from build123d import *

# Parameters (mm, degrees)
SKETCH1_W               = 177.8
SKETCH1_H               = 25.4
BOSS_EXTRUDE1_DEPTH     = 4.826
SKETCH2_W               = 46.566666667
SKETCH2_H               = 4.826
SKETCH2_W_2             = 46.566666666
BOTTOM_EDGE_SLOTS_DEPTH = 180.669948172
SKETCH3_W               = 79.375
SKETCH3_H               = 4.826
TOP_EDGE_SLOTS_DEPTH    = 180.669948172
SKETCH4_W               = 4.826
SKETCH4_H               = 15.748
EDGE_CUTS_DEPTH         = 180.669948172


with BuildPart() as part:
    # Sketch1 → Boss-Extrude1 (new body)
    with BuildSketch(Plane.XY):
        with Locations((88.9, 12.7)):
            Rectangle(SKETCH1_W, SKETCH1_H)
    extrude(amount=BOSS_EXTRUDE1_DEPTH)

    # Sketch2 → Bottom Edge Slots (cut, through all)
    with BuildSketch(Plane.XY.offset(4.826)):
        with Locations((23.283333333, 2.413)):
            Rectangle(SKETCH2_W, SKETCH2_H)
        with Locations((88.9, 2.413)):
            Rectangle(SKETCH2_W_2, SKETCH2_H)
        with Locations((154.516666667, 2.413)):
            Rectangle(SKETCH2_W, SKETCH2_H)
    extrude(amount=-BOTTOM_EDGE_SLOTS_DEPTH, mode=Mode.SUBTRACT)

    # Sketch3 → Top Edge Slots (cut, through all)
    with BuildSketch(Plane.XY.offset(4.826)):
        with Locations((39.6875, 22.987)):
            Rectangle(SKETCH3_W, SKETCH3_H)
        with Locations((138.1125, 22.987)):
            Rectangle(SKETCH3_W, SKETCH3_H)
    extrude(amount=-TOP_EDGE_SLOTS_DEPTH, mode=Mode.SUBTRACT)

    # Sketch4 → Edge Cuts (cut, through all)
    with BuildSketch(Plane.XY.offset(4.826)):
        with Locations((2.413, 12.7)):
            Rectangle(SKETCH4_W, SKETCH4_H)
        with Locations((175.387, 12.7)):
            Rectangle(SKETCH4_W, SKETCH4_H)
    extrude(amount=-EDGE_CUTS_DEPTH, mode=Mode.SUBTRACT)


solid = part.part
Design review of the part built by this model. Coordinates are the model's own, in mm. A direction names the side the tool comes from. Give positions to 0.01 mm unless a question says otherwise; leave off trailing zeros. Order: outer loops, then holes, each group sorted by start corner. A loop starts at its lowest first (then second) coordinate and runs counter-clockwise, first axis right, second up.
1. Mouldability with a two-part tool opening along X and no side actions: class faces 1 (the flat face through (131.233, 2, 2)), 2 (the flat face through (56, 0, 2)), 3 (the flat face through (65.617, 2, 2)) as +X half, -X half, draft (parallel to the pull), parting line (faces both ways), or undercut.
Solution:
face 1: +X half
face 2: draft
face 3: undercut
2. Add section C-C, the plane y = 23.25. State the section outline as (x, z) points (3 decimals), then the cut area to 3 significant figures.
Solution:
outline: (79.375, 0) - (98.425, 0) - (98.425, 4.826) - (79.375, 4.826) - close
area: 91.9 mm2
3. To check wall thickness, follow L1, parallel to X at y = 4.25, z = 0.4; L2, parallel to Y at x = 128.5, z = 0.2; L3, parallel to Y at x = 22, z = 2.75. State the ranges of each line that lie inside material, in increasing order.
Solution:
L1: x = 46.57 to 65.62, 112.18 to 131.23
L2: y = 0 to 20.57
L3: y = 4.83 to 20.57
4. Add section B-B, the plane x = 101. State the section outline as (y, z) points, then the cut area to 3 significant figures.
Solution:
outline: (4.83, 0) - (20.57, 0) - (20.57, 4.83) - (4.83, 4.83) - close
area: 76.0 mm2
5. For pin 1 Ø4 at (x, y) = (105, 17.5) entering from -Z; pin 2 Ø1.4 at (x, z) = (143.5, 3) entering from +Y; pin 3 Ø2.5 at (y, z) = (1.5, 1.5) entering from -X; pin 4 Ø1.4 at (x, z) = (20.5, 2) entering from -Y, all flat-tipped, find the tip position at first contact; note any pin that passes through.
Solution:
pin 1: stops at z = 0
pin 2: stops at y = 20.57
pin 3: stops at x = 46.57
pin 4: stops at y = 4.83
6. Tool access review of faces 4 (the flat face through (152, 4.826, 2)), 5 (the flat face through (135, 20.574, 2)), 6 (the flat face through (79.375, 23, 2)): name each direction out of +Z, -Z, +X, -X, +Y, -Y from which nothing blocks a thin tool from reaching the whole face with its end or side.
Solution:
face 4: +Z, -Z, +X, -Y
face 5: +Z, -Z, +X, +Y
face 6: +Z, -Z, -X, +Y
7. Add section A-A, the plane z = 1.4. State the section outline as (x, y) points (3 decimals), then the cut area to 3 significant figures.
Solution:
outline: (4.826, 4.826) - (46.567, 4.826) - (46.567, 0) - (65.617, 0) - (65.617, 4.826) - (112.183, 4.826) - (112.183, 0) - (131.233, 0) - (131.233, 4.826) - (172.974, 4.826) - (172.974, 20.574) - (98.425, 20.574) - (98.425, 25.4) - (79.375, 25.4) - (79.375, 20.574) - (4.826, 20.574) - close
area: 2,920 mm2
